Autodesk Inventor part; units mm, degrees
sketch "スケッチ1" plane through (0, 0, 0) normal (0, 0, 1) x (1, 0, 0)
  arc A0 (0, 100) -> (0, -100) centre (0, 0) ccw
  line L0 (0, 100) -> (0, -100)
  dimension "d0" = 200
revolve "回転1" add sketch "スケッチ1" angle 360 about axis through (0, 100, 0) along (0, -1, 0)
ref_plane "作業平面1" through (0, 0, 300) normal (0, 0, 1) x (1, 0, 0)
ref_plane "作業平面2" through (0, 100, 0) normal (0, 1, 0) x (-1, 0, 0)
ref_plane "作業平面3" through (0, -100, 0) normal (0, 1, 0) x (-1, 0, 0)
ref_plane "作業平面4" through (0, 0, 100) normal (0, 0, 1) x (1, 0, 0)
sketch "スケッチ2" plane through (0, 0, 0) normal (1, 0, 0) x (0, 1, 0)
  line L0 (134.8667, -67.7722) -> (-130.8003, -67.7722)
  line L1 (-130.8003, -67.7722) -> (-130.8003, -136.448)
  line L2 (-130.8003, -136.448) -> (134.8667, -136.448)
  line L3 (134.8667, -136.448) -> (134.8667, -67.7722)
  point P0 (0, 0)
extrude "押し出し1" cut sketch "スケッチ2" along normal mid plane 200
sketch "スケッチ3" plane through (0, 0, 0) normal (0, 1, 0) x (-1, 0, 0)
  circle A0 centre (0, 0) radius 25
  dimension "d8" = 50
extrude "押し出し2" cut sketch "スケッチ3" along normal mid plane 200
sketch "スケッチ4" plane through (0, 0, 0) normal (0, 0, 1) x (1, 0, 0)
  circle A0 centre (0, 0) radius 25
  dimension "d11" = 50
extrude "押し出し3" add sketch "スケッチ4" along normal blind 200
sketch "スケッチ5" plane through (0, 0, 0) normal (0, 1, 0) x (-1, 0, 0)
  circle A0 centre (0, 100) radius 25
  point P0 (0, 0)
  dimension "d14" = 50
  dimension "d15" = 100
extrude "押し出し4" add sketch "スケッチ5" along normal mid plane 100
properties part number "ChestP"
Check sheet for the modelled part. Datum: model origin and axes. Units: mm. A direction names the side the tool comes from. Round coordinates to 2 decimals unless told otherwise and drop trailing zeros. Loops run counter-clockwise (first coordinate to the right, second up) from the corner with the lowest first, then second, coordinate; pieces in that order, holes last. Notation, with made-up numbers: (48, 43.5) -> (58, 43.5) arc R22 cw to (58, 78.5) -> close; hole circle Ø6 at (11, 54). An arc over 180 degrees is marked (long way). Answer in a Markdown table with one row per item.
Q1. Thickness scan on L1, parallel to Z at x = 0, y = -7; L2, parallel to Z at x = 0, y = -33; L3, parallel to X at y = 56, z = 0. Record the ranges inside material, lowest first.
Data:
| item | result |
|---|---|
| L1 | z = -67.77 to -25, 0 to 200 |
| L2 | z = -67.77 to -25, 25 to 125 |
| L3 | x = -82.85 to -25, 25 to 82.85 |
Q2. Sectioned sample at B-B on y = -8. Enter the section's corners in (x, z) (1 decimal).
Data:
| item | result |
|---|---|
| outline | (-73.1, -67.8) -> (73.1, -67.8) arc R99.7 ccw to (24.8, 96.6) arc R25 ccw to (23.7, 108) -> (23.7, 200) -> (-23.7, 200) -> (-23.7, 108) arc R25 ccw to (-24.8, 96.6) arc R99.7 ccw to start; hole (-23.7, 0) -> (-23.7, 8) arc R25 ccw (long way) to (23.7, 8) -> (23.7, 0) -> close |
Q3. Sectioned sample at D-D on x = -48.5. Enter the section's corners in (y, z).
Data:
| item | result |
|---|---|
| outline | (-55.27, -67.77) -> (55.27, -67.77) arc R87.45 ccw (long way) to start |
Q4. Release check for a two-part mould opening along Z. For faces 3 (the face through (0, 0, 200)), 4 (the face through (3.255, -1.356, -24.787)), 5 (the face through (-20, 15, 160)), 6 (the face through (-0.55, 24.994, 9.58)) record: released by +Z, released by -Z, zero draft, split by the parting line, or undercut.
Data:
| item | result |
|---|---|
| face 3 | released by +Z |
| face 4 | undercut |
| face 5 | zero draft |
| face 6 | undercut |
Q5. Sectioned sample at C-C on z = 136. Enter the section's corners in (x, y), then the cut area to 3 significant figures.
Data:
| item | result |
|---|---|
| outline | circle Ø50 at (0, 0) |
| area | 1,960 mm^2 |
Q6. Go/stop test with flat-tipped pins: P1, Ø4, axis at x = 18.5, z = 144, coming from the +Y side; P2, Ø1, axis at x = -57.5, y = 46.5, coming from the +Z side; P3, Ø8, axis at x = 44.5, z = -18.5, coming from the +Y side. Record where each tip stops, or that it passes through.
Data:
| item | result |
|---|---|
| P1 | stops at y = 18.78 |
| P2 | stops at z = 67.86 |
| P3 | stops at y = 89.71 |
Q7. Set-up check for faces 1 (the face through (-1, 1, -67.772)), 2 (the face through (0, 0, 0)): record each of +Z, -Z, +X, -X, +Y, -Y from which the full face is reachable in a straight line by a thin tool's end or side.
Data:
| item | result |
|---|---|
| face 1 | -Z, +X, -X, +Y, -Y |
| face 2 | +Y, -Y |
Q8. Sectioned sample at A-A on x = 0. Enter the section's corners in (y, z), then the cut area to 3 significant figures.
Data:
| item | result |
|---|---|
| outline | (-96.82, -25) arc R100 ccw to (-73.53, -67.77) -> (73.53, -67.77) arc R100 ccw to (96.82, -25) -> close; (-96.82, 25) -> (-25, 25) -> (-25, 0) -> (25, 0) -> (25, 25) -> (96.82, 25) arc R100 ccw to (50, 86.6) -> (50, 125) -> (25, 125) -> (25, 200) -> (-25, 200) -> (-25, 125) -> (-50, 125) -> (-50, 86.6) arc R100 ccw to start |
| area | 26,200 mm^2 |
